Design review of the part built by this model. Coordinates are the model's own, in mm. A direction names the side the tool comes from. Coordinates: 2 decimals unless noted, no trailing zeros. Write each loop counter-clockwise with the first axis right and the second up, starting at its lowest first coordinate (ties: lowest second). Pieces come first, ordered by that corner, then holes.
Q1. Take a section at A-A (z = 9). Give the boundary of the cut face in (x, y) (3 decimals).
Q2. Mouldability with a two-part tool opening along X and no side actions: class faces 1 (the flat face through (-7, 3.175, -3)), 2 (the flat face through (-7, -3.175, -3)), 3 (the flat face through (-546.88, 36.25, -3.2)), 4 (the flat face through (543.41, 41.76, 3.2)) as pulls with the +X half, pulls with the -X half, needs draft (parallel to the pull), parting line crosses it, or undercut.
Q3. Insertion check: pin 1 (3 mm diameter, centred on y = 15.5, z = -139, fed in from -X); pin 2 (8 mm diameter, centred on y = 10.5, z = 126.5, fed in from -X); pin 3 (1.5 mm diameter, centred on y = 8.5, z = -181.5, fed in from +X). Each pin has a flat end and moves straight along its axis. Give the tip position at first contact, or say it passes through.
Q4. Take a section at B-B (x = -317.5). Give the boundary of the cut face in (y, z) (3 decimals).
Q5. For probe 1 along Y at (x, z) = (376, 198) (3 decimals); probe 2 along X at (y, z) = (54, -76.5); probe 3 along X at (y, z) = (57, 46), list the stretches that pass through material, from the lowest coordinate up.
Q6. Machinability: for faces 5 (the flat face through (-543.41, 41.76, -3.2)), 6 (the flat face through (546.88, 36.25, 3.2)), which of the approach directions +Z, -Z, +X, -X, +Y, -Y give a long, thin tool a straight path to every point of the face, cutting with its end or side? Answer none if there is none.
```python
from build123d import *

# Parameters (mm, degrees)
BASE_FLANGE1_START             = -3.175
BASE_FLANGE1_OUTLINE_W         = 1009.65
BASE_FLANGE1_OUTLINE_H         = 457.2
BASE_FLANGE1_DEPTH             = 6.35
EDGE_FLANGE1_STRIP_CUT_DEPTH   = 457.2
EDGE_FLANGE1_STRIP_CUT_2_DEPTH = 457.2
EDGE_FLANGE1_DEPTH             = 457.2
EDGE_FLANGE1_BEND_DEPTH        = 457.2
SKETCH12_R                     = 9.525
CUT_EXTRUDE1_DEPTH             = 6.35
SKETCH13_R                     = 9.525
CUT_EXTRUDE2_DEPTH             = 6.35


# Read off the part's stored shape, not the designer's step: Base-Flange1
# Sheet-metal steps are written as plain solids
with BuildPart() as part:
    # Base-Flange1 outline → Base-Flange1 (new body)
    with BuildSketch(Plane(origin=(0, 0, 0), x_dir=(1, 0, 0), z_dir=(0, 1, 0)).offset(BASE_FLANGE1_START)):
        Rectangle(BASE_FLANGE1_OUTLINE_W, BASE_FLANGE1_OUTLINE_H)
    extrude(amount=BASE_FLANGE1_DEPTH)

    # Edge-Flange1 strip (across the edge) → Edge-Flange1 strip cut (cut)
    with BuildSketch(Plane(origin=(504.825, 3.175, 228.6), x_dir=(-0.7071067811865438, 0.7071067811865512, 0), z_dir=(0, 0, -1))):
        Polygon((-29.571024484, 20.590768363), (-2.630256121, -6.35), (1.859871939, -1.859871939), (-25.080896424, 25.080896424), align=None)
    extrude(amount=EDGE_FLANGE1_STRIP_CUT_DEPTH, mode=Mode.SUBTRACT)

    # Edge-Flange1 strip 2 (across the edge) → Edge-Flange1 strip cut 2 (cut)
    with BuildSketch(Plane(origin=(-504.825, 3.175, -228.6), x_dir=(0.7071067811865438, 0.7071067811865512, 0), z_dir=(0, 0, 1))):
        Polygon((-29.571024484, 20.590768363), (-2.630256121, -6.35), (1.859871939, -1.859871939), (-25.080896424, 25.080896424), align=None)
    extrude(amount=EDGE_FLANGE1_STRIP_CUT_2_DEPTH, mode=Mode.SUBTRACT)

    # Edge-Flange1 section (across the edge) → Edge-Flange1 (add)
    with BuildSketch(Plane(origin=(504.825, 3.175, 228.6), x_dir=(-0.7071067811865438, 0.7071067811865512, 0), z_dir=(0, 0, -1))):
        with BuildLine():
            Line((-6.35, 2.630256121), (-6.35, 105.065743879))
            Line((-6.35, 105.065743879), (0, 105.065743879))
            Line((0, 105.065743879), (0, 2.630256121))
            ThreePointArc((0, 2.630256121), (0.483364969, 0.200216326), (1.859871939, -1.859871939))
            Line((1.859871939, -1.859871939), (-2.630256121, -6.35))
            ThreePointArc((-2.630256121, -6.35), (-5.383270063, -2.22982347), (-6.35, 2.630256121))
        make_face()
    extrude(amount=EDGE_FLANGE1_DEPTH)

    # Edge-Flange1 section 2 (across the edge) → Edge-Flange1 bend (add)
    with BuildSketch(Plane(origin=(-504.825, 3.175, -228.6), x_dir=(0.7071067811865438, 0.7071067811865512, 0), z_dir=(0, 0, 1))):
        with BuildLine():
            Line((-6.35, 2.630256121), (-6.35, 105.065743879))
            Line((-6.35, 105.065743879), (0, 105.065743879))
            Line((0, 105.065743879), (0, 2.630256121))
            ThreePointArc((0, 2.630256121), (0.483364969, 0.200216326), (1.859871939, -1.859871939))
            Line((1.859871939, -1.859871939), (-2.630256121, -6.35))
            ThreePointArc((-2.630256121, -6.35), (-5.383270063, -2.22982347), (-6.35, 2.630256121))
        make_face()
    extrude(amount=EDGE_FLANGE1_BEND_DEPTH)

    # Sketch12 → Cut-Extrude1 (cut)
    with BuildSketch(Plane(origin=(255.315128061, -255.315128061, 0), x_dir=(-0.7071067811865513, -0.7071067811865438, 0), z_dir=(0.7071067811865438, -0.7071067811865513, 0))):
        with Locations(Location((-410.427988722, -206.375, 0), (0, 0, 180))):
            Circle(SKETCH12_R)
        with Locations(Location((-410.427988722, 206.375, 0), (0, 0, 180))):
            Circle(SKETCH12_R)
    extrude(amount=-CUT_EXTRUDE1_DEPTH, mode=Mode.SUBTRACT)

    # Sketch13 → Cut-Extrude2 (cut)
    with BuildSketch(Plane(origin=(-255.315128061, -255.315128061, 0), x_dir=(0, 0, 1), z_dir=(-0.7071067811865442, -0.7071067811865509, 0))):
        with Locations(Location((-206.375, 410.427988722, 0), (0, 0, 270))):
            Circle(SKETCH13_R)
        with Locations(Location((206.375, 410.427988722, 0), (0, 0, 90))):
            Circle(SKETCH13_R)
    extrude(amount=-CUT_EXTRUDE2_DEPTH, mode=Mode.SUBTRACT)


solid = part.part
```
Response:
1. outline: (-583.608, 72.978) - (-511.175, 0.545) arc R12.7 ccw to (-502.195, -3.175) - (502.195, -3.175) arc R12.7 ccw to (511.175, 0.545) - (583.608, 72.978) - (579.118, 77.468) - (506.685, 5.035) arc R6.35 cw to (502.195, 3.175) - (-502.195, 3.175) arc R6.35 cw to (-506.685, 5.035) - (-579.118, 77.468) - close
2. face 1: undercut
2. face 2: needs draft
2. face 3: pulls with the -X half
2. face 4: undercut
3. pin 1: stops at x = -527.63
3. pin 2: stops at x = -525.13
3. pin 3: stops at x = 519.88
4. outline: (-3.175, -228.6) - (3.175, -228.6) - (3.175, 228.6) - (-3.175, 228.6) - close
5. probe 1: y = -3.175 to 3.175
5. probe 2: x = -564.63 to -555.65, 555.65 to 564.63
5. probe 3: x = -567.63 to -558.65, 558.65 to 567.63
6. face 5: +Z, -Z, +Y
6. face 6: +Z, -Z, +X, -Y
